from build123d import *

# Parameters (mm, degrees)
F1_DEPTH      = 38.1
F1_DEPTH_BACK = 38.1
F2_R          = 7.8493938986
F2_R_2        = 6.2054902318
F3_DEPTH      = 76.201
F4_W          = 44.9225585908
F4_H          = 36.150701344
F4_H_2        = 55.2893020213
F5_DEPTH      = 43.0628599057
F6_R          = 6.2054902318
F7_DEPTH      = 60.95999991


with BuildPart() as f1:
    # F0 (on Right) → F1 (new body, two sides)
    with BuildSketch(Plane.YZ) as f1_sk:
        with BuildLine():
            Line((-21.5309299529, 32.9609289765), (-21.5309299529, -22.3283730447))
            ThreePointArc((-21.5309299529, -22.3283730447), (0, -43.8593029976), (21.5309299529, -22.3283730447))
            Line((21.5309299529, -22.3283730447), (21.5309299529, 32.9609289765))
            ThreePointArc((21.5309299529, 32.9609289765), (0, 54.4918589294), (-21.5309299529, 32.9609289765))
        make_face()
    extrude(amount=F1_DEPTH)
    extrude(f1_sk.sketch, amount=-F1_DEPTH_BACK)

    # F2 (on face) → F3 (cut, through all)
    with BuildSketch(Plane.YZ.offset(38.1)):
        with Locations((0, 32.9609289765)):
            Circle(F2_R)
        with Locations((0, -22.3283730447)):
            Circle(F2_R_2)
    extrude(amount=-F3_DEPTH, mode=Mode.SUBTRACT)

    # F4 (on face) → F5 (cut, through all)
    with BuildSketch(Plane(origin=(0, 21.5309299529, 0), x_dir=(-1, 0, 0), z_dir=(0, 1, 0))):
        with Locations((0.3987206146, 51.0362796485)):
            Rectangle(F4_W, F4_H)
        with Locations((0.3987206146, 5.3162779659)):
            Rectangle(F4_W, F4_H_2)
    extrude(amount=-F5_DEPTH, mode=Mode.SUBTRACT)

    # F6 (on face) → F7 (join, through all)
    with BuildSketch(Plane.YZ.offset(-22.85999991)):
        with BuildLine():
            ThreePointArc((21.5309299529, -22.3283730447), (0, -0.7974430919), (-21.5309299529, -22.3283730447))
            ThreePointArc((-21.5309299529, -22.3283730447), (0, -43.8593029976), (21.5309299529, -22.3283730447))
        make_face()
        with Locations((0, -22.3283730447)):
            Circle(F6_R, mode=Mode.SUBTRACT)
    extrude(amount=F7_DEPTH)


solid = f1.part
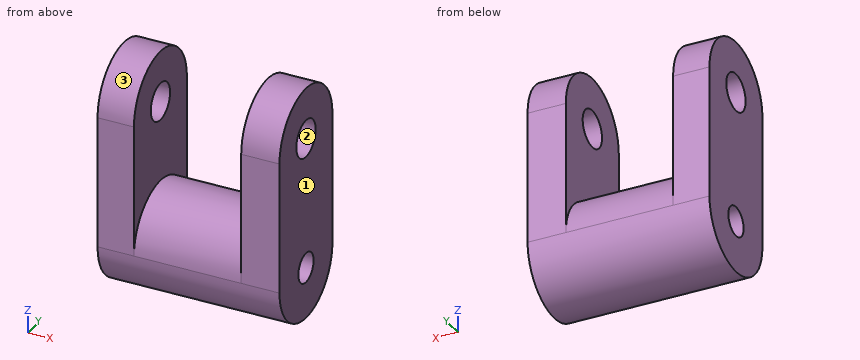
Model file for the job. Use its own axes, mm. Face numbers are marked on the shaded views. Give positions to 0.01 mm unless a question says otherwise; leave off trailing zeros. Loops run counter-clockwise (first coordinate to the right, second up) from the corner with the lowest first, then second, coordinate; pieces in that order, holes last.
Item 1: Slice it at D-D (x = 13.5). Write the cut outline in (y, z), plus the area to 3 significant figures.
Check values:
outline: circle Ø43.06 at (0, -22.33); hole circle Ø12.41 at (0, -22.33)
area: 1,340 mm2
Item 2: Slice it at C-C (x = 30.5). Write the cut outline in (y, z), plus the area to 3 significant figures.
Check values:
outline: (-21.53, -22.33) arc R21.53 ccw to (21.53, -22.33) - (21.53, 32.96) arc R21.53 ccw to (-21.53, 32.96) - close; hole circle Ø15.7 at (0, 32.96); hole circle Ø12.41 at (0, -22.33)
area: 3,520 mm2
Item 3: Drill centre lines: line 1 along Z through (x, y) = (27, 0); line 2 along X through (y, z) = (9.5, 36.5); line 3 along Y through (x, z) = (29, 32.5). Where is each one in solid material? Low to high.
Check values:
line 1: z = -43.86 to -28.53, -16.12 to 25.11, 40.81 to 54.49
line 2: x = -38.1 to -22.86, 22.06 to 38.1
line 3: y = -21.53 to -7.84, 7.84 to 21.53
Item 4: Slice it at B-B (z = 16.5). Write the cut outline in (x, y).
Check values:
outline: (-38.1, -21.53) - (-22.86, -21.53) - (-22.86, 21.53) - (-38.1, 21.53) - close; (22.06, -21.53) - (38.1, -21.53) - (38.1, 21.53) - (22.06, 21.53) - close
Item 5: Drop flat-ended pins along their axis: P1, Ø10, axis at x = 5, y = -1, coming from the +Z side; P2, Ø10, axis at x = 23.5, y = -15.5, coming from the -Z side; P3, Ø1, axis at x = 27.5, z = 39, coming from the -Y side. Give the stop position or say it passes through.
Check values:
P1: stops at z = -0.8
P2: stops at z = -41.13
P3: stops at y = -20.81
Item 6: Mould opens along Z. For the marked faces 1, 2 and 3 say: +Z half, -Z half, draft (parallel to the pull), parting line (faces both ways), or undercut.
Check values:
face 1: draft
face 2: undercut
face 3: +Z half
Item 7: Slice it at A-A (y = 0). Write the cut outline in (x, z), plus the area to 3 significant figures.
Check values:
outline: (-38.1, -43.86) - (38.1, -43.86) - (38.1, -28.53) - (-38.1, -28.53) - close; (-38.1, -16.12) - (38.1, -16.12) - (38.1, 25.11) - (22.06, 25.11) - (22.06, -0.8) - (-22.86, -0.8) - (-22.86, 25.11) - (-38.1, 25.11) - close; (-38.1, 40.81) - (-22.86, 40.81) - (-22.86, 54.49) - (-38.1, 54.49) - close; (22.06, 40.81) - (38.1, 40.81) - (38.1, 54.49) - (22.06, 54.49) - close
area: 3,570 mm2
